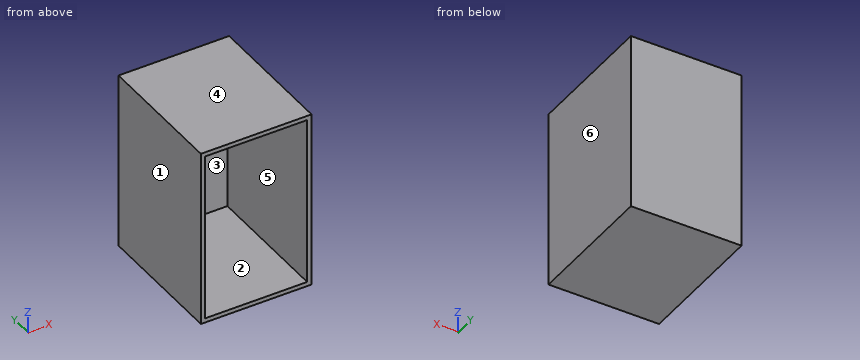
```python
from build123d import *

# Parameters (mm, degrees)
F0_W     = 298.3636856079
F0_H     = 497.2105026245
F1_DEPTH = 381
F2_T     = 12.7


with BuildPart() as f1:
    # F0 (on Front) → F1 (new body)
    with BuildSketch(Plane.XZ):
        Rectangle(F0_W, F0_H)
    extrude(amount=F1_DEPTH)

    # F2
    f2_openings = [f1.faces().sort_by_distance(p)[0] for p in [
        (0, -381, 0),
    ]]
    offset(amount=F2_T, openings=f2_openings, kind=Kind.INTERSECTION)


solid = f1.part
```
The listing builds one solid part. Answer for the finished solid, in the listing's coordinates (mm). Face numbers are marked on the shaded views. A direction names the side the tool comes from. Give positions to 0.01 mm unless a question says otherwise; leave off trailing zeros. Write each loop counter-clockwise with the first axis right and the second up, starting at its lowest first coordinate (ties: lowest second). Pieces come first, ordered by that corner, then holes. Notation, with made-up numbers: (-22.5, -20) -> (-18.5, -20) arc R20 ccw to (-18.5, 5) -> close; hole circle Ø9 at (23, -37.75). An arc over 180 degrees is marked (long way). Write item = value, one per line. Start each with the question number.
1) The part is cut by section B-B, the plane x = 113.5. Determine the outline of the cut face in (y, z), and give its area (3 significant figures).
2) Which of the six approach directions +Z, -Z, +X, -X, +Y, -Y give full straight-line access (tool end or side, diameter ignored) to the marked faces 1 and 2?
3) Straight lines are drawn through the part: line 1 along Z through (x, y) = (0.5, -10.5); line 2 along X through (y, z) = (-97.5, -45); line 3 along Y through (x, z) = (-130, 31.5). For each, find the intervals that lie inside material, in ascending order.
4) The part is cut by section C-C, the plane z = -163.5. Determine the outline of the cut face in (x, y).
5) This flat-tipped pin is pushed along its axis until it touches: pin 1 (6 mm diameter, centred on x = 62.5, z = 178.5, fed in from -Y). Where does it stop, or does it pass through?
6) The part is cut by section A-A, the plane y = -198. Determine the outline of the cut face in (x, z), and give its area (3 significant figures).
7) Determine the mould class of the marked faces 3, 4, 5 and 6 for opening direction X: +X half, -X half, draft (parallel to the pull), parting line (faces both ways), or undercut.
Solutions:
q1.outline = (-381, -261.31) -> (12.7, -261.31) -> (12.7, 261.31) -> (-381, 261.31) -> (-381, 248.61) -> (0, 248.61) -> (0, -248.61) -> (-381, -248.61) -> close
q1.area = 16,300 mm²
q2.face_1 = +Z, -Z, -X, +Y, -Y
q2.face_2 = -Y
q3.line_1 = -261.31 to -248.61, 248.61 to 261.31
q3.line_2 = -161.88 to -149.18, 149.18 to 161.88
q3.line_3 = 0 to 12.7
q4.outline = (-161.88, -381) -> (-149.18, -381) -> (-149.18, 0) -> (149.18, 0) -> (149.18, -381) -> (161.88, -381) -> (161.88, 12.7) -> (-161.88, 12.7) -> close
q5.pin_1 = 0
q6.outline = (-161.88, -261.31) -> (161.88, -261.31) -> (161.88, 261.31) -> (-161.88, 261.31) -> close; hole (-149.18, -248.61) -> (149.18, -248.61) -> (149.18, 248.61) -> (-149.18, 248.61) -> close
q6.area = 20,900 mm²
q7.face_3 = undercut
q7.face_4 = draft
q7.face_5 = undercut
q7.face_6 = +X half
